from build123d import *

# Parameters (mm, degrees)
BOSS_EXTRUDE1_OUTLINE_R = 1.75
BOSS_EXTRUDE1_DEPTH     = 4
CUT_EXTRUDE1_DEPTH      = 1


# Read off the part's stored shape, not the designer's step: Boss-Extrude1
with BuildPart() as part:
    # Boss-Extrude1 outline → Boss-Extrude1 (new body)
    with BuildSketch(Plane(origin=(0, 0, 0), x_dir=(1, 0, 0), z_dir=(0, 1, 0))):
        with BuildLine():
            Line((25.416474615, -10.33744254), (37.24307775, -10.33744254))
            ThreePointArc((37.24307775, -10.33744254), (39.679776182, -5.587442326), (42.116474615, -10.33744254))
            Line((42.116474615, -10.33744254), (49.179776182, -10.33744254))
            Line((49.179776182, -10.33744254), (49.179776182, -18.81631662))
            Line((49.179776182, -18.81631662), (58.804776182, -18.81631662))
            Line((58.804776182, -18.81631662), (58.804776182, -4.977921711))
            Line((58.804776182, -4.977921711), (-21.195223818, -4.977921711))
            Line((-21.195223818, -4.977921711), (-21.195223818, -18.81631662))
            Line((-21.195223818, -18.81631662), (-11.570223818, -18.81631662))
            Line((-11.570223818, -18.81631662), (-11.570223818, -10.33744254))
            Line((-11.570223818, -10.33744254), (3.84307775, -10.33744254))
            ThreePointArc((3.84307775, -10.33744254), (6.279776182, -5.587442326), (8.716474615, -10.33744254))
            Line((8.716474615, -10.33744254), (20.54307775, -10.33744254))
            ThreePointArc((20.54307775, -10.33744254), (22.979776182, -5.587442326), (25.416474615, -10.33744254))
        make_face()
        with Locations((-16.195223818, -13.587442433)):
            Circle(BOSS_EXTRUDE1_OUTLINE_R, mode=Mode.SUBTRACT)
        with Locations((53.804776182, -13.587442433)):
            Circle(BOSS_EXTRUDE1_OUTLINE_R, mode=Mode.SUBTRACT)
    extrude(amount=BOSS_EXTRUDE1_DEPTH)

    # Sketch2 → Cut-Extrude1 (cut)
    # profile 1 of 2: a face of its own
    with BuildSketch(Plane(origin=(0, 4, 0), x_dir=(1, 0, 0), z_dir=(0, 1, 0))):
        Polygon((-16.41198232, -6.812466594), (-14.865187448, -6.812466594), (-14.865187448, -7.382338389), (-15.842110525, -7.382338389), (-15.842110525, -7.992915312), (-14.865187448, -7.992915312), (-14.865187448, -8.562787107), (-15.842110525, -8.562787107), (-15.842110525, -9.987466594), (-16.41198232, -9.987466594), align=None)
    # profile 2 of 2: a face of its own
    with BuildSketch(Plane(origin=(0, 4, 0), x_dir=(1, 0, 0), z_dir=(0, 1, 0))):
        with BuildLine():
            Line((-13.509197865, -10.06887685), (-14.014195862, -9.814469799))
            Line((-14.014195862, -9.814469799), (-13.460860525, -8.725607619))
            add(Edge.make_bspline(
                [(-13.460860525, -8.725607619), (-13.493552847, -8.724774336), (-13.557735785, -8.723138398), (-13.652240154, -8.70954377), (-13.742612406, -8.686336872), (-13.829917734, -8.655442645), (-13.912948731, -8.614025733), (-13.992712215, -8.564596821), (-14.068103991, -8.505208694), (-14.139477538, -8.438453984), (-14.204643867, -8.364668422), (-14.261206862, -8.285313298), (-14.310508019, -8.20240162), (-14.348847302, -8.114061596), (-14.37964161, -8.021939666), (-14.402141484, -7.925558996), (-14.414767818, -7.82449673), (-14.416532622, -7.755714857), (-14.417431038, -7.720699767)],
                knots=[0, 0, 0, 0, 1.014336294, 1.991387562, 2.955278539, 3.906441712, 4.859855302, 5.829322156, 6.813833455, 7.833278715, 8.858926674, 9.863225732, 10.85404919, 11.846815163, 12.845559416, 13.865450493, 14.913355531, 16, 16, 16, 16], degree=3))
            add(Edge.make_bspline(
                [(-14.417431038, -7.720699767), (-14.416597708, -7.686735475), (-14.414955648, -7.619809541), (-14.40131818, -7.521584049), (-14.378874437, -7.427273226), (-14.348082426, -7.336893095), (-14.307090423, -7.251053103), (-14.259110328, -7.168409197), (-14.200456838, -7.09067119), (-14.134198348, -7.017502553), (-14.061681947, -6.950566169), (-13.984748133, -6.89171273), (-13.903746713, -6.84251691), (-13.819718635, -6.801201496), (-13.73114503, -6.77033319), (-13.639305886, -6.747043281), (-13.543517063, -6.733601675), (-13.478497608, -6.731911573), (-13.445596102, -6.731056337)],
                knots=[0, 0, 0, 0, 1.055538678, 2.079917126, 3.075849687, 4.065898488, 5.041806164, 6.028602842, 7.031727914, 8.062953097, 9.093756959, 10.095582084, 11.068815425, 12.035667573, 13.000833448, 13.979119574, 14.977382875, 16, 16, 16, 16], degree=3))
            add(Edge.make_bspline(
                [(-13.445596102, -6.731056337), (-13.411193598, -6.731764476), (-13.343545729, -6.733156934), (-13.244518332, -6.748522162), (-13.149772928, -6.772095231), (-13.058924549, -6.804112269), (-12.97310104, -6.847566016), (-12.891584275, -6.899645635), (-12.814645404, -6.96150342), (-12.743110693, -7.03135644), (-12.678050673, -7.107334669), (-12.620383061, -7.186865545), (-12.571939818, -7.269793563), (-12.532261839, -7.355378619), (-12.501352894, -7.443754793), (-12.480106932, -7.535047442), (-12.466001971, -7.629100452), (-12.464397107, -7.692875343), (-12.463584884, -7.72515189)],
                knots=[0, 0, 0, 0, 1.062826075, 2.08990367, 3.089830715, 4.078784409, 5.060762809, 6.057138927, 7.064407536, 8.107320944, 9.143871033, 10.153461498, 11.140480137, 12.108246174, 13.065926856, 14.029354859, 15.002654194, 16, 16, 16, 16], degree=3))
            add(Edge.make_bspline(
                [(-12.463584884, -7.72515189), (-12.464028122, -7.749768446), (-12.464920902, -7.799351725), (-12.473699398, -7.873707226), (-12.487018143, -7.94826881), (-12.502477367, -8.01095661), (-12.518684213, -8.063798617), (-12.534455319, -8.108625261), (-12.554690113, -8.158391252), (-12.577284282, -8.213430161), (-12.60345099, -8.273500634), (-12.633732754, -8.338315513), (-12.666299428, -8.408836066), (-12.690304282, -8.45705706), (-12.702727513, -8.482012868)],
                knots=[0, 0, 0, 0, 1.105131805, 2.225983929, 3.357782449, 4.505488967, 5.122909461, 5.839607681, 6.638776516, 7.535249922, 8.51168636, 9.581005249, 10.748097757, 12, 12, 12, 12], degree=3))
            Line((-12.702727513, -8.482012868), (-13.509197865, -10.06887685))
        make_face()
        with BuildLine():
            add(Edge.make_bspline(
                [(-13.43287575, -8.196440953), (-13.405569868, -8.194833376), (-13.352220356, -8.191692536), (-13.275587332, -8.16740689), (-13.207004671, -8.125847553), (-13.146217368, -8.07063542), (-13.095984603, -8.003274093), (-13.059462095, -7.92658921), (-13.036965354, -7.84216883), (-13.034648703, -7.783384123), (-13.033456679, -7.753136666)],
                knots=[0, 0, 0, 0, 0.984774978, 1.924027336, 2.867853169, 3.859505234, 4.871392407, 5.881338128, 6.909850265, 8, 8, 8, 8], degree=3))
            add(Edge.make_bspline(
                [(-13.033456679, -7.753136666), (-13.034892342, -7.722259992), (-13.03768505, -7.66219749), (-13.0603973, -7.575750698), (-13.099207968, -7.497607925), (-13.152007661, -7.429680335), (-13.213650613, -7.37283362), (-13.282582994, -7.331308626), (-13.357130982, -7.305630901), (-13.408720798, -7.302506546), (-13.434783803, -7.300928132)],
                knots=[0, 0, 0, 0, 1.104110315, 2.147758178, 3.172670271, 4.206310416, 5.210906102, 6.157051016, 7.068948237, 8, 8, 8, 8], degree=3))
            add(Edge.make_bspline(
                [(-13.434783803, -7.300928132), (-13.462330936, -7.302466882), (-13.516419507, -7.305488204), (-13.594004346, -7.331104267), (-13.665525389, -7.371831843), (-13.72798309, -7.428871436), (-13.782037835, -7.495904441), (-13.819731685, -7.574310981), (-13.843578121, -7.660154514), (-13.846208342, -7.720324727), (-13.847559243, -7.751228613)],
                knots=[0, 0, 0, 0, 0.970967322, 1.90648639, 2.855811969, 3.858352357, 4.877096915, 5.878517833, 6.91039038, 8, 8, 8, 8], degree=3))
            add(Edge.make_bspline(
                [(-13.847559243, -7.751228613), (-13.846148143, -7.781691987), (-13.8434037, -7.840940069), (-13.820402477, -7.92583923), (-13.782935789, -8.002929935), (-13.731716155, -8.070822503), (-13.668626178, -8.126306671), (-13.596992367, -8.167423317), (-13.517086507, -8.191758387), (-13.461451298, -8.194852), (-13.43287575, -8.196440953)],
                knots=[0, 0, 0, 0, 1.075706617, 2.092137047, 3.084482865, 4.090466434, 5.0784141, 6.035155512, 6.990809768, 8, 8, 8, 8], degree=3))
        make_face(mode=Mode.SUBTRACT)
    extrude(amount=-CUT_EXTRUDE1_DEPTH, mode=Mode.SUBTRACT)


solid = part.part
Design review of the part built by this model. Coordinates are the model's own, in mm. A direction names the side the tool comes from. Coordinates: 2 decimals unless noted, no trailing zeros. Order: outer loops, then holes, each group sorted by start corner. A loop starts at its lowest first (then second) coordinate and runs counter-clockwise, first axis right, second up. Notation, with made-up numbers: M 56.5,-24.5 L 90.5,-24.5 A8 cw 90.5,-11.5 Z; hole C 82,78.5 d2. An arc over 180 degrees is marked long. Use a Markdown table: item, result.
(1) Add section A-A (z = 18). Give the boundary of the cut face in (x, y).
Worked answers:
| item | result |
|---|---|
| outline | M -21.2,0 L -11.57,0 L -11.57,4 L -21.2,4 Z; M 49.18,0 L 58.8,0 L 58.8,4 L 49.18,4 Z |
(2) Draft analysis for pull direction X (two halves, no side actions). For faces 3 (the flat face through (-16, 2, 18.816)), 4 (the flat face through (-13.4, 3, 8.4)), 5 (the flat face through (-21.195, 2, 12)), state which applies: released by +X, released by -X, zero draft, split by the parting line, or undercut.
Worked answers:
| item | result |
|---|---|
| face 3 | zero draft |
| face 4 | undercut |
| face 5 | released by -X |
(3) Add section B-B (x = 54). Give the boundary of the cut face in (y, z), then the cut area to 3 significant figures.
Worked answers:
| item | result |
|---|---|
| outline | M 0,4.98 L 4,4.98 L 4,11.85 L 0,11.85 Z; M 0,15.33 L 4,15.33 L 4,18.82 L 0,18.82 Z |
| area | 41.4 mm2 |
(4) Add section D-D (z = 12.5). Give the boundary of the cut face in (x, y).
Worked answers:
| item | result |
|---|---|
| outline | M -21.2,0 L -17.57,0 L -17.57,4 L -21.2,4 Z; M -14.82,0 L -11.57,0 L -11.57,4 L -14.82,4 Z; M 49.18,0 L 52.43,0 L 52.43,4 L 49.18,4 Z; M 55.18,0 L 58.8,0 L 58.8,4 L 55.18,4 Z |
(5) For faces 1 (the flat face through (19, 2, 4.978)), 2 (the flat face through (15, 2, 10.337)), list the 3-axis set-ups (+Z, -Z, +X, -X, +Y, -Y) from which the entire face can be reached by the end or side of a thin tool; tool diameter is ignored.
Worked answers:
| item | result |
|---|---|
| face 1 | -Z, +X, -X, +Y, -Y |
| face 2 | +Z, +Y, -Y |
(6) For P1, Ø1, axis at x = 48.5, y = 1.5, coming from the +Z side, flat-tipped, find the tip position at first contact; note if it passes through.
Worked answers:
| item | result |
|---|---|
| P1 | stops at z = 10.34 |
(7) Wall thickness on probe 1 along X at (y, z) = (1.65, 14); probe 2 along X at (y, z) = (0.2, 9.5); probe 3 along X at (y, z) = (2.3, 16.75): over which ranges is each line inside the solid? List them lowest first.
Worked answers:
| item | result |
|---|---|
| probe 1 | x = -21.2 to -17.9, -14.49 to -11.57, 49.18 to 52.1, 55.51 to 58.8 |
| probe 2 | x = -21.2 to 3.42, 9.14 to 20.12, 25.84 to 36.82, 42.54 to 58.8 |
| probe 3 | x = -21.2 to -11.57, 49.18 to 58.8 |
(8) Add section C-C (y = 1.6). Give the boundary of the cut face in (x, z), then the cut area to 3 significant figures.
Worked answers:
| item | result |
|---|---|
| outline | M -21.2,4.98 L 58.8,4.98 L 58.8,18.82 L 49.18,18.82 L 49.18,10.34 L 42.12,10.34 A3 cw long 37.24,10.34 L 25.42,10.34 A3 cw long 20.54,10.34 L 8.72,10.34 A3 cw long 3.84,10.34 L -11.57,10.34 L -11.57,18.82 L -21.2,18.82 Z; hole C -16.2,13.59 d3.5; hole C 53.8,13.59 d3.5 |
| area | 501 mm2 |
